Answer from the drawing. Dimensions are ordinates in mm from the lowest x, y and z of the part. A direction names the side the tool comes from. Coordinates: 2 decimals unless noted, no trailing zeros. Loops run counter-clockwise (first coordinate to the right, second up) from the corner with the lowest first, then second, coordinate; pieces in that order, holes last. Notation, with made-up numbers: (69.25, -18) -> (122.25, -18) arc R17 ccw to (122.25, -11) -> close; hole circle Ø1 at (73, 43.5). An arc over 180 degrees is marked (long way). Answer as CSV lines item,"result".
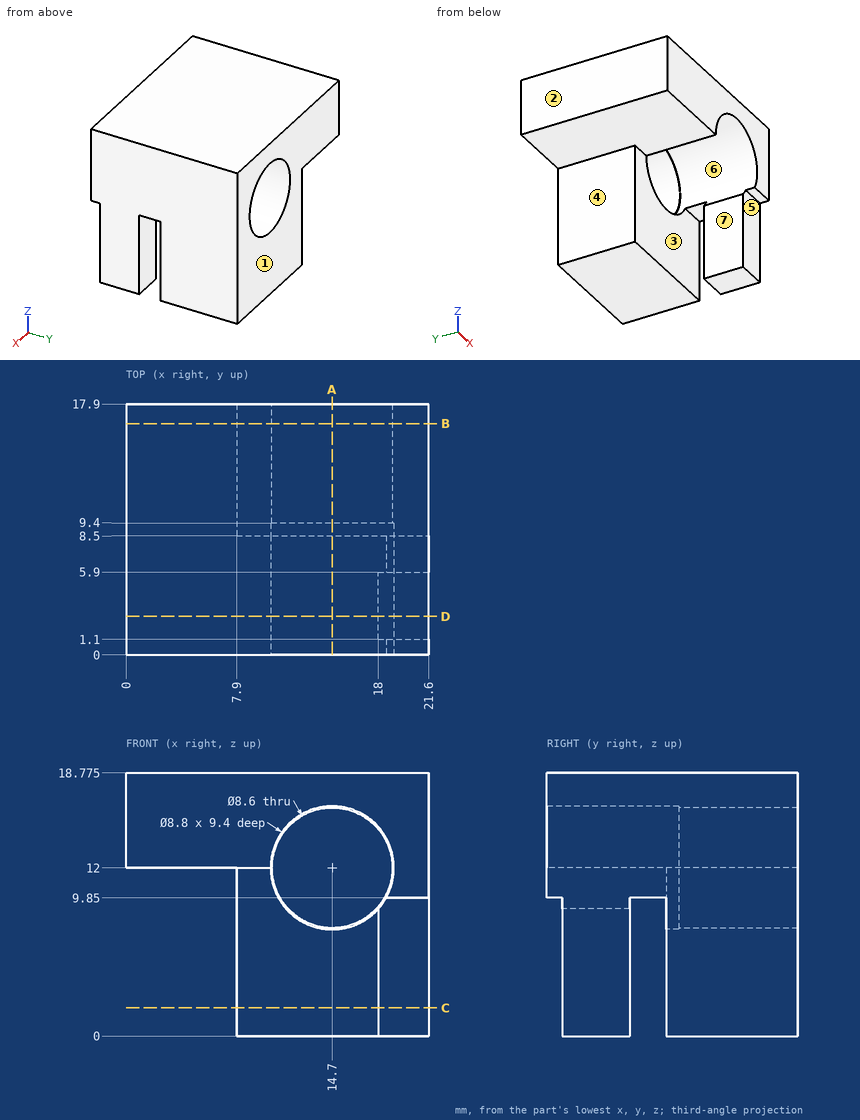
(1) Which of the six approach directions +Z, -Z, +X, -X, +Y, -Y give full straight-line access (tool end or side, diameter ignored) to the marked faces 4, 5, 6 and 7?
Computed values:
face 4,"-Z, -X, +Y, -Y"
face 5,"-Z, +X, -X, -Y"
face 6,"-Y"
face 7,"-Z, -X, -Y"
(2) For a pull along Y with two mould halves and no side action, classify the marked faces 1, 2 and 3 as pulls with the +Y half, pulls with the -Y half, needs draft (parallel to the pull), parting line crosses it, or undercut.
Computed values:
face 1,"pulls with the +Y half"
face 2,"needs draft"
face 3,"undercut"
(3) Flat-ended cylindrical pins translate along their axes: pin 1 Ø7.5 at (y, z) = (14.5, 5) entering from -X; pin 2 Ø3.5 at (x, z) = (13.5, 3) entering from -Y; pin 3 Ø8 at (x, y) = (3.5, 5) entering from -Z. Find the tip coordinate at first contact, or state that the pin passes through.
Computed values:
pin 1,"x = 7.9"
pin 2,"y = 8.5"
pin 3,"z = 12"
(4) A cutting plane is placed at D-D, the plane y = 2.75. Write down the section's boundary in (x, z) (3 decimals), and give its area (3 significant figures).
Computed values:
outline,"(0, 12) -> (10.3, 12) arc R4.4 cw (long way) to (18, 9.09) -> (18, 0) -> (21.6, 0) -> (21.6, 18.775) -> (0, 18.775) -> close"
area,"157 mm2"
(5) A cutting plane is placed at A-A, the plane x = 14.7. Write down the section's boundary in (y, z) (3 decimals).
Computed values:
outline,"(0, 16.4) -> (9.4, 16.4) -> (9.4, 16.3) -> (17.9, 16.3) -> (17.9, 18.775) -> (0, 18.775) -> close; (8.5, 0) -> (17.9, 0) -> (17.9, 7.7) -> (9.4, 7.7) -> (9.4, 7.6) -> (8.5, 7.6) -> close"
(6) A cutting plane is placed at B-B, the plane y = 16.5. Write down the section's boundary in (x, z) (3 decimals).
Computed values:
outline,"(0, 12) -> (7.9, 12) -> (7.9, 0) -> (21.6, 0) -> (21.6, 18.775) -> (0, 18.775) -> close; hole circle Ø8.6 at (14.7, 12)"
(7) A cutting plane is placed at C-C, the plane z = 2. Write down the section's boundary in (x, y), and give its area (3 significant figures).
Computed values:
outline,"(7.9, 8.5) -> (21.6, 8.5) -> (21.6, 17.9) -> (7.9, 17.9) -> close; (18, 1.1) -> (21.6, 1.1) -> (21.6, 5.9) -> (18, 5.9) -> close"
area,"146 mm2"
(8) Consider line 1 along Z through (x, y) = (14.7, 15.75) (3 decimals); line 2 along Y through (x, z) = (20.5, 4.75); line 3 along Z through (x, y) = (2.75, 6) (3 decimals). Determine where each line is inside the solid, lowest interval first.
Computed values:
line 1,"0 to 7.7, 16.3 to 18.775"
line 2,"1.1 to 5.9, 8.5 to 17.9"
line 3,"12 to 18.775"
